from build123d import *

# Parameters (mm, degrees)
SKETCH1_R           = 12.7
BOSS_EXTRUDE1_DEPTH = 51.816
FILLET1_R           = 1
SKETCH2_R           = 9.017
BOSS_EXTRUDE3_DEPTH = 9.53
SKETCH5_R           = 5.4991
CUT_EXTRUDE1_DEPTH  = 50.8
SKETCH6_R           = 2.3495
CUT_EXTRUDE2_DEPTH  = 50.8


with BuildPart() as part:
    # Sketch1 → Boss-Extrude1 (new body)
    with BuildSketch(Plane.XY):
        Circle(SKETCH1_R)
    extrude(amount=BOSS_EXTRUDE1_DEPTH)

    # Fillet1
    fillet1_edges = [part.edges().sort_by_distance(p)[0] for p in [
        (-12.7, 0, 0),
        (-12.7, 0, 51.816),
    ]]
    fillet(fillet1_edges, radius=FILLET1_R)

    # Sketch2 → Boss-Extrude3 (add)
    with BuildSketch(Plane.XY.offset(51.816)):
        Circle(SKETCH2_R)
    extrude(amount=BOSS_EXTRUDE3_DEPTH)

    # Sketch5 → Cut-Extrude1 (cut)
    with BuildSketch(Plane(origin=(0, 0, 0), x_dir=(-1, 0, 0), z_dir=(0, 0, -1))):
        Circle(SKETCH5_R)
    extrude(amount=-CUT_EXTRUDE1_DEPTH, mode=Mode.SUBTRACT)

    # Sketch6 → Cut-Extrude2 (cut)
    with BuildSketch(Plane.XY.offset(61.346)):
        Circle(SKETCH6_R)
    extrude(amount=-CUT_EXTRUDE2_DEPTH, mode=Mode.SUBTRACT)


solid = part.part
Work out the finished part from the listing and answer in its coordinate system (mm). A direction names the side the tool comes from. Give positions to 0.01 mm unless a question says otherwise; leave off trailing zeros. Loops run counter-clockwise (first coordinate to the right, second up) from the corner with the lowest first, then second, coordinate; pieces in that order, holes last. Notation, with made-up numbers: (-13, 12) - (45, 12) arc R20 cw to (45, 41) - close; hole circle Ø8 at (-35.75, 61). An arc over 180 degrees is marked (long way). Answer in a Markdown table with one row per item.
(1) Flat-ended cylindrical pins translate along their axes: pin 1 Ø5.5 at (x, y) = (0, -0.5) entering from -Z; pin 2 Ø6 at (x, z) = (-7, 32.5) entering from +Y; pin 3 Ø6 at (x, y) = (-8.5, 6) entering from -Z; pin 4 Ø10 at (x, z) = (-8.5, 38) entering from +Y. Find the tip coordinate at first contact, or state that the pin passes through.
Results list:
| item | result |
|---|---|
| pin 1 | stops at z = 50.8 |
| pin 2 | stops at y = 12.05 |
| pin 3 | stops at z = 0 |
| pin 4 | stops at y = 12.21 |
(2) For a pull along Y with two mould halves and no side action, classify faces 1 (the face through (-1.955, -8.803, 56.514)), 2 (the face through (6, -7, 51.816)), 3 (the face through (-0.31, 2.33, 56.15)) as pulls with the +Y half, pulls with the -Y half, needs draft (parallel to the pull), parting line crosses it, or undercut.
Results list:
| item | result |
|---|---|
| face 1 | parting line crosses it |
| face 2 | needs draft |
| face 3 | undercut |
(3) A tool of negligible diameter and unlimited length cuts with its end or side. For faces 4 (the face through (2, -2, 61.346)), 5 (the face through (-2.4, -1.1, 50.8)), from which of +Z, -Z, +X, -X, +Y, -Y can it reach the whole face along a straight path? Write none if from no direction.
Results list:
| item | result |
|---|---|
| face 4 | +Z, +X, -X, +Y, -Y |
| face 5 | -Z |
(4) Consider L1, parallel to Y at x = 0, z = 40; L2, parallel to Y at x = -1.5, z = 32; L3, parallel to Z at x = 11.25, y = 2.75. Determine where each line is inside the solid, lowest interval first. Write a range as [from, to].
Results list:
| item | result |
|---|---|
| L1 | y = [-12.7, -5.5], [5.5, 12.7] |
| L2 | y = [-12.61, -5.29], [5.29, 12.61] |
| L3 | z = [0, 51.82] |
(5) Section C-C (z = 46) is taken. Give the vertices of the cut face in (x, y).
Results list:
| item | result |
|---|---|
| outline | circle Ø25.4 at (0, 0); hole circle Ø11 at (0, 0) |
(6) Section A-A (y = 0) is taken. Give the vertices of the cut face in (x, z), and give its area (3 significant figures).
Results list:
| item | result |
|---|---|
| outline | (-12.7, 1) arc R1 ccw to (-11.7, 0) - (-5.5, 0) - (-5.5, 50.8) - (-2.35, 50.8) - (-2.35, 61.35) - (-9.02, 61.35) - (-9.02, 51.82) - (-11.7, 51.82) arc R1 ccw to (-12.7, 50.82) - close; (2.35, 50.8) - (5.5, 50.8) - (5.5, 0) - (11.7, 0) arc R1 ccw to (12.7, 1) - (12.7, 50.82) arc R1 ccw to (11.7, 51.82) - (9.02, 51.82) - (9.02, 61.35) - (2.35, 61.35) - close |
| area | 879 mm² |
